from build123d import *

# Parameters (mm, degrees)
F1_R     = 15.875
F3_R     = 12.2021545383
F4_DEPTH = 50.8


with BuildPart() as f2:
    # F2: sweep along a path in F0
    with BuildLine(Plane.XZ) as f2_path:
        Line((-344.3413384318, -41.1043575529), (550.2936645415, -41.1043575529))
        ThreePointArc((550.2936645415, -41.1043575529), (645.2322257553, -7.9202524438), (698.826283108, 77.1808183703))
        Line((698.826283108, 77.1808183703), (842.452537594, 702.5155299205))
        Line((842.452537594, 702.5155299205), (-735.4231768463, 0))
        Line((-735.4231768463, 0), (-344.3413384318, -41.1043575529))
    # F1 (on Right) → F2 (sweep)
    with BuildSketch(Plane.YZ):
        with Locations((0, -41.1043575529)):
            Circle(F1_R)
    sweep(path=f2_path.line, transition=Transition.RIGHT)

    # F3 (on Front) → F4 (join)
    with BuildSketch(Plane.XZ):
        with Locations((-636.8260383606, 15.446998179)):
            Circle(F3_R)
    extrude(amount=-F4_DEPTH)


solid = f2.part
Part model, mm, in its own coordinate system. Coordinates: 2 decimals unless noted, no trailing zeros. Order: outer loops, then holes, each group sorted by start corner. A loop starts at its lowest first (then second) coordinate and runs counter-clockwise, first axis right, second up. Notation, with made-up numbers: M -31,21 L 7,21 A19 cw 7,58 Z; hole C -32,64 d11. An arc over 180 degrees is marked long. One line per question, with ' | ' between items.
Q1. Slice it at A-A (y = 32). Give the cut face in (x, z), and give its area (3 significant figures).
A:
outline: C -636.83,15.45 d24.4 | area: 468 mm^2
Q2. Drill centre lines: line 1 (X direction, y = -8, z = 140); line 2 (Z direction, x = -390.5, y = 5.5); line 3 (Z direction, x = 105.5, y = -3.5). Where is each one in solid material? Low to high.
A:
line 1: x = -454.69 to -387.27, 699.19 to 727.32 | line 2: z = -51.23 to -21.28, 137.27 to 169.87 | line 3: z = -56.59 to -25.62, 357.45 to 391.35
Q3. Pin check, flat tips, straight feed: P1, Ø12, axis at y = 7, z = 211, coming from the +X side; P2, Ø5, axis at x = -507, y = 15, coming from the -Z side; P3, Ø10, axis at y = -4, z = 283.5, coming from the -X side. Stop position of each tip, or through.
A:
P1: stops at x = 746.58 | P2: stops at z = -33.86 | P3: stops at x = -148
